from build123d import *

# Parameters (mm, degrees)
SKETCH3_R           = 40
BOSS_EXTRUDE4_DEPTH = 3
SKETCH6_R           = 1.5
SKETCH6_R_2         = 8.75
CUT_EXTRUDE2_DEPTH  = 165.951508026
CHAMFER1_SIZE       = 1.5
SKETCH12_W          = 2
SKETCH12_H          = 10
BOSS_EXTRUDE7_DEPTH = 10
SKETCH13_R          = 1.25
CUT_EXTRUDE8_DEPTH  = 180.357185527
SKETCH14_R          = 2.5
CUT_EXTRUDE9_DEPTH  = 166.435788148
CHAMFER2_SIZE       = 3
CUT_EXTRUDE10_DEPTH = 166.435788148
FILLET1_R           = 5


with BuildPart() as part:
    # Sketch3 → Boss-Extrude4 (new body)
    with BuildSketch(Plane.XY):
        with BuildLine():
            ThreePointArc((40, 0), (0, 40), (-40, 0))
            Line((-40, 0), (40, 0))
        make_face()
        with BuildLine():
            Line((40, 0), (-40, 0))
            ThreePointArc((-40, 0), (0, -40), (40, 0))
        make_face()
        with BuildLine():
            Line((-40, 120), (-40, 0))
            ThreePointArc((-40, 0), (0, 40), (40, 0))
            Line((40, 0), (40, 120))
            ThreePointArc((40, 120), (0, 80), (-40, 120))
        make_face()
        with Locations((0, 120)):
            Circle(SKETCH3_R)
    extrude(amount=BOSS_EXTRUDE4_DEPTH)

    # Sketch6 → Cut-Extrude2 (cut, through all)
    with BuildSketch(Plane(origin=(0, 0, 0), x_dir=(-1, 0, 0), z_dir=(0, 0, -1))):
        with Locations((-7.5, 29.007101127)):
            Circle(SKETCH6_R)
        with Locations((7.5, 29.007101127)):
            Circle(SKETCH6_R)
        with Locations((0, -16.25)):
            Circle(SKETCH6_R)
        Circle(SKETCH6_R_2)
    extrude(amount=-CUT_EXTRUDE2_DEPTH, mode=Mode.SUBTRACT)

    # Chamfer1
    chamfer1_edges = [part.edges().sort_by_distance(p)[0] for p in [
        (-6, 29.007101127, 3),
        (1.5, -16.25, 3),
        (9, 29.007101127, 3),
    ]]
    chamfer(chamfer1_edges, length=CHAMFER1_SIZE)

    # Sketch12 → Boss-Extrude7 (add)
    with BuildSketch(Plane.XY.offset(3)):
        with Locations((39, 115)):
            Rectangle(SKETCH12_W, SKETCH12_H)
        with Locations((-39, 115)):
            Rectangle(SKETCH12_W, SKETCH12_H)
        with Locations((-39, 5)):
            Rectangle(SKETCH12_W, SKETCH12_H)
        with Locations((39, 5)):
            Rectangle(SKETCH12_W, SKETCH12_H)
    extrude(amount=BOSS_EXTRUDE7_DEPTH)

    # Sketch13 → Cut-Extrude8 (cut, through all)
    with BuildSketch(Plane.ZY.offset(40)):
        with Locations((8, 115)):
            Circle(SKETCH13_R)
        with Locations((8, 5)):
            Circle(SKETCH13_R)
    extrude(amount=-CUT_EXTRUDE8_DEPTH, mode=Mode.SUBTRACT)

    # Sketch14 → Cut-Extrude9 (cut, through all)
    with BuildSketch(Plane(origin=(0, 0, 0), x_dir=(-1, 0, 0), z_dir=(0, 0, -1))):
        with Locations((-21, 21.5)):
            Circle(SKETCH14_R)
        with Locations((21, 21.5)):
            Circle(SKETCH14_R)
    extrude(amount=-CUT_EXTRUDE9_DEPTH, mode=Mode.SUBTRACT)

    # Chamfer2
    chamfer2_edges = [part.edges().sort_by_distance(p)[0] for p in [
        (23.5, 21.5, 0),
        (-18.5, 21.5, 0),
    ]]
    chamfer(chamfer2_edges, length=CHAMFER2_SIZE - 0.0001)  # a hair under: the kernel refuses the full size

    # Sketch9 → Cut-Extrude10 (cut, through all)
    with BuildSketch(Plane(origin=(0, 0, 0), x_dir=(-1, 0, 0), z_dir=(0, 0, -1))):
        with BuildLine():
            ThreePointArc((3, 40), (0, 43), (-3, 40))
            Line((-3, 40), (-3, 24))
            ThreePointArc((-3, 24), (0, 15), (3, 24))
            Line((3, 24), (3, 40))
        make_face()
    extrude(amount=-CUT_EXTRUDE10_DEPTH, mode=Mode.SUBTRACT)

    # Fillet1
    fillet1_edges = [part.edges().sort_by_distance(p)[0] for p in [
        (3, 24, 1.5),
        (-3, 24, 1.5),
    ]]
    fillet(fillet1_edges, radius=FILLET1_R)


solid = part.part
For this review, take the finished solid that the model builds, in its own axes (mm). A direction names the side the tool comes from. Round coordinates to 2 decimals unless told otherwise and drop trailing zeros. Order: outer loops, then holes, each group sorted by start corner. A loop starts at its lowest first (then second) coordinate and runs counter-clockwise, first axis right, second up. Notation, with made-up numbers: (7.5, 13) -> (31.5, 13) arc R5 cw to (31.5, 22) -> close; hole circle Ø6 at (9, 57). An arc over 180 degrees is marked (long way). Put each result on its own line as item: value.
Q1. Insertion check: pin 1 Ø1.5 at (x, z) = (-12, 4) entering from +Y; pin 2 Ø1.6 at (x, z) = (-39, 7.5) entering from +Y; pin 3 Ø8 at (x, y) = (12, 23.5) entering from +Z; pin 4 Ø2 at (x, z) = (-39.5, 10) entering from -Y. Each pin has a flat end and moves straight along its axis. Give the tip position at first contact, or say it passes through.
Check result:
pin 1: through
pin 2: y = 120
pin 3: z = 3
pin 4: y = 0
Q2. Machinability: for faces 4 (the flat face through (-38, 6, 9)), 5 (the flat face through (-40, 61, 2)), which of the approach directions +Z, -Z, +X, -X, +Y, -Y give a long, thin tool a straight path to every point of the face, cutting with its end or side? Answer none if there is none.
Check result:
face 4: +Z, +Y, -Y
face 5: +Z, -Z, -X, +Y, -Y
Q3. For probe 1 along Y at (x, z) = (-39.6, 8); probe 2 along Z at (x, y) = (28, -1.5); probe 3 along X at (y, z) = (-13.5, 1.25), list the stretches that pass through material, from the lowest coordinate up. Write a range as [from, to].
Check result:
probe 1: [0, 3.75], [6.25, 10], [110, 113.75], [116.25, 120]
probe 2: [0, 3]
probe 3: [-37.65, 37.65]
Q4. Add section B-B on y = 37.5. Write out the cut boundary in (x, z), plus the area to 3 significant figures.
Check result:
outline: (-40, 0) -> (-3, 0) -> (-3, 3) -> (-40, 3) -> close; (3, 0) -> (40, 0) -> (40, 3) -> (3, 3) -> close
area: 222 mm2
Q5. Mouldability with a two-part tool opening along X and no side actions: class faces 1 (the cylindrical face through (0.88, 159.99, 1.48)), 2 (the flat face through (40, 59, 2)), 3 (the flat face through (38, 114, 9)) as pulls with the +X half, pulls with the -X half, needs draft (parallel to the pull), parting line crosses it, or undercut.
Check result:
face 1: parting line crosses it
face 2: pulls with the +X half
face 3: undercut
Q6. Add section A-A on z = 4.75. Write out the cut boundary in (x, y), plus the area to 3 significant figures.
Check result:
outline: (-40, 0) -> (-38, 0) -> (-38, 10) -> (-40, 10) -> close; (-40, 110) -> (-38, 110) -> (-38, 120) -> (-40, 120) -> close; (38, 0) -> (40, 0) -> (40, 10) -> (38, 10) -> close; (38, 110) -> (40, 110) -> (40, 120) -> (38, 120) -> close
area: 80.0 mm2
Q7. Add section D-D on y = 98. Write out the cut boundary in (x, z).
Check result:
outline: (-40, 0) -> (40, 0) -> (40, 3) -> (-40, 3) -> close
